Autodesk Inventor part; units mm, degrees
ref_plane "Work Plane1" through (-9, 0, 0) normal (0, 0, -1) x (0, 1, 0)
ref_plane "YZ Plane" through (0, 0, 0) normal (1, 0, 0) x (0, 1, 0)
ref_plane "XZ Plane" through (0, 0, 0) normal (0, 1, 0) x (-1, 0, 0)
sketch "Sketch1" plane through (0, 0, 0) normal (0, 1, 0) x (-1, 0, 0)
  circle A0 centre (0, 0) radius 13.5
  line L0 (0, 0) -> (9, 0)
  line L1 (0, 0) -> (-9, 0)
  circle A1 centre (-9, 0) radius 2
  circle A2 centre (9, 0) radius 2
  dimension "d0" = 27
  dimension "d1" = 9
  dimension "d2" = 9
  dimension "d3" = 4
  dimension "d4" = 4
extrude "Extrusion1" add sketch "Sketch1" along normal blind 5
sketch "Sketch2" plane through (0, 5, 0) normal (0, 1, 0) x (1, 0, 0)
  circle A0 centre (0, 0) radius 25
  circle A1 centre (-9, 0) radius 2
  circle A2 centre (9, 0) radius 2
  circle A3 centre (-9, 0) radius 2
  circle A4 centre (-9, 0) radius 2
  circle A5 centre (9, 0) radius 2
  circle A6 centre (9, 0) radius 2
  dimension "d7" = 50
extrude "Extrusion2" add sketch "Sketch2" along normal blind 6
sketch "Sketch3" plane through (0, 11, 0) normal (0, 1, 0) x (1, 0, 0)
  circle A0 centre (0, 0) radius 28.5
  circle A1 centre (-9, 0) radius 2
  circle A2 centre (9, 0) radius 2
  circle A3 centre (-9, 0) radius 2
  circle A4 centre (9, 0) radius 2
  circle A5 centre (9, 0) radius 2
  dimension "d10" = 57
extrude "Extrusion4" add sketch "Sketch3" along normal blind 1.5
ref_plane "Work Plane1" through (-9, 0, 0) normal (0, 0, -1) x (0, 1, 0)
sketch "Sketch4" plane through (-9, 0, 0) normal (0, 0, -1) x (0, 1, 0)
  line L0 (0, 9) -> (5, 9)
  line L1 (5, -4.5) -> (5, 22.5)
  circle A0 centre (2.5, 9) radius 1.5
  dimension "d15" = 3
extrude "Extrusion5" cut sketch "Sketch4" against normal up to surface
properties part number "Wrist-Bearing Attachment"
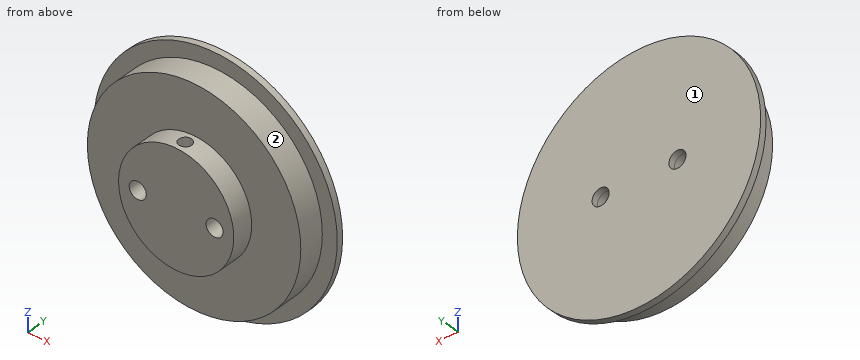
For this review, take the finished solid that the model builds, in its own axes (mm). Face numbers are marked on the shaded views. A direction names the side the tool comes from. Coordinates: 2 decimals unless noted, no trailing zeros. Write each loop counter-clockwise with the first axis right and the second up, starting at its lowest first coordinate (ties: lowest second). Pieces come first, ordered by that corner, then holes.
(1) Tool access review of the marked faces 1 and 2: name each direction out of +Z, -Z, +X, -X, +Y, -Y from which nothing blocks a thin tool from reaching the whole face with its end or side.
(2) Add section C-C on y = 7. Give the boundary of the cut face in (x, z).
(3) For pin 1 Ø1 at (x, z) = (19.5, 22) entering from -Y; pin 2 Ø5 at (x, y) = (1, 9.5) entering from -Z; pin 3 Ø4 at (y, z) = (8.5, -14) entering from +X; pin 4 Ø4 at (x, y) = (3, 6) entering from -Z, all flat-tipped, find the tip position at first contact; note any pin that passes through.
(4) Add section A-A on z = 6. Give the boundary of the cut face in (x, y), then the cut area to 3 significant figures.
(5) Wall thickness on probe 1 along X at (y, z) = (11.4, 0); probe 2 along X at (y, z) = (8.5, 0); probe 3 along Y at (x, z) = (20.5, 14.5): over which ranges is each line inside the solid? List them lowest first.
(6) Add section B-B on x = 0. Give the boundary of the cut face in (y, z), then the cut area to 3 significant figures.
(7) Add section D-D on z = 17. Give the boundary of the cut face in (x, y), then the cut area to 3 significant figures.
Answer sheet:
1. face 1: +Z, -Z, +X, -X, +Y
1. face 2: -Y
2. outline: circle Ø50 at (0, 0); hole circle Ø4 at (-9, 0); hole circle Ø4 at (9, 0)
3. pin 1: passes through
3. pin 2: stops at z = -28.5
3. pin 3: stops at x = 21.93
3. pin 4: stops at z = -24.98
4. outline: (-27.86, 11) - (-24.27, 11) - (-24.27, 5) - (-12.09, 5) - (-12.09, 0) - (12.09, 0) - (12.09, 5) - (24.27, 5) - (24.27, 11) - (27.86, 11) - (27.86, 12.5) - (-27.86, 12.5) - close; hole circle Ø3 at (0, 2.5)
4. area: 489 mm2
5. probe 1: x = -28.5 to -11, -7 to 7, 11 to 28.5
5. probe 2: x = -25 to -11, -7 to 7, 11 to 25
5. probe 3: y = 11 to 12.5
6. outline: (0, -13.5) - (5, -13.5) - (5, -25) - (11, -25) - (11, -28.5) - (12.5, -28.5) - (12.5, 28.5) - (11, 28.5) - (11, 25) - (5, 25) - (5, 13.5) - (4, 13.5) - (4, 0) - (1, 0) - (1, 13.5) - (0, 13.5) - close
6. area: 480 mm2
7. outline: (-22.87, 11) - (-18.33, 11) - (-18.33, 5) - (18.33, 5) - (18.33, 11) - (22.87, 11) - (22.87, 12.5) - (-22.87, 12.5) - close
7. area: 289 mm2
